Can you work these out from the model? Positions are in its coordinate system, mm. Face numbers are marked on the shaded views. A direction names the side the tool comes from. Round coordinates to 2 decimals unless told otherwise and drop trailing zeros. Write each loop counter-clockwise with the first axis right and the second up, starting at its lowest first coordinate (ties: lowest second). Pieces come first, ordered by that corner, then holes. Notation, with made-up numbers: M 89.5,56.25 L 112.5,56.25 A22 ccw 112.5,93.25 Z; hole C 33,56.25 d4. An arc over 180 degrees is marked long. Answer in a Markdown table with one row per item. Add a question column.
(1) Suppose I cut it at A-A, the plane x = 25. Write out the boundary of the cut face in (y, z) (3 decimals).
(2) If we mould it in two halves opening along X, with no side actions, what happens to the marked faces 1, 2 and 3? For each: released by +X, released by -X, zero draft, split by the parting line, or undercut.
(3) I'm going to push flat-ended pins straight in: pin 1 (5 mm diameter, centred on y = 2.5, z = 14.5, fed in from -X); pin 2 (8 mm diameter, centred on x = 25.5, z = 13.5, fed in from -Y); pin 3 (5 mm diameter, centred on y = 4.5, z = 7, fed in from -X); pin 4 (2 mm diameter, centred on x = 21, y = 2.5, fed in from +Z). Where does each tip first touch, or does it pass through?
(4) For the marked faces 4 and 5, which set-ups out of +Z, -Z, +X, -X, +Y, -Y let a thin tool reach every point of the face, with its end or its side?
(5) Suppose I cut it at B-B, the plane z = 16.75. Write out the boundary of the cut face in (x, y), then the cut area to 3 significant figures.
(6) Suppose I cut it at D-D, the plane z = 1.5. Write out the boundary of the cut face in (x, y) (3 decimals).
(7) If I drill on probe 1 along Y at (x, z) = (25, 3.25) (3 decimals); probe 2 along Z at (x, y) = (25, 0.45); probe 3 along X at (y, z) = (6.75, 18), over which ranges is the centre line in solid material (lowest first)?
(8) Suppose I cut it at C-C, the plane y = 4.25. Write out the boundary of the cut face in (x, z), then the cut area to 3 significant figures.
from build123d import *

# Parameters (mm, degrees)
PAD001_DEPTH = 1
PAD012_DEPTH = 10
SKETCH012_R  = 1.475
POCKET_DEPTH = 50


with BuildPart() as part:
    # Sketch001 → Pad001 (new body)
    with BuildSketch(Plane.XZ):
        with BuildLine():
            ThreePointArc((17.153982, 21), (25, 9.6), (32.846018, 21))
            Line((36.846018, 21), (32.846018, 21))
            Line((50, 0), (36.846018, 21))
            Line((0, 0), (50, 0))
            Line((13.153982, 21), (0, 0))
            Line((17.153982, 21), (13.153982, 21))
        make_face()
    extrude(amount=-PAD001_DEPTH)

    # Sketch011 → Pad012 (join)
    with BuildSketch(Plane.XZ):
        with BuildLine():
            ThreePointArc((14.157376, 21), (25, 6.75), (35.842624, 21))
            Line((40.842624, 21), (35.842624, 21))
            Line((50, 0), (40.842624, 21))
            Line((0, 0), (50, 0))
            Line((9.157376, 21), (0, 0))
            Line((14.157376, 21), (9.157376, 21))
        make_face()
    extrude(amount=-PAD012_DEPTH)

    # Sketch012 → Pocket (cut)
    with BuildSketch(Plane.XY):
        with Locations((25, 5)):
            Circle(SKETCH012_R)
    extrude(amount=POCKET_DEPTH, mode=Mode.SUBTRACT)


solid = part.part
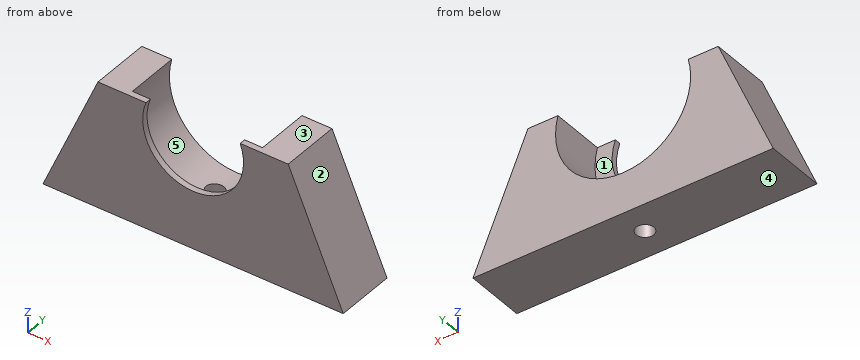
Calculated:
| question | item | result |
|---|---|---|
| 1 | outline | M 0,0 L 3.525,0 L 3.525,6.75 L 1,6.75 L 1,9.6 L 0,9.6 Z; M 6.475,0 L 10,0 L 10,6.75 L 6.475,6.75 Z |
| 2 | face 1 | undercut |
| 2 | face 2 | released by +X |
| 2 | face 3 | zero draft |
| 3 | pin 1 | x = 5.23 |
| 3 | pin 2 | y = 0 |
| 3 | pin 3 | x = 1.96 |
| 3 | pin 4 | z = 7.92 |
| 4 | face 4 | -Z, +X, -X, +Y, -Y |
| 4 | face 5 | +Y |
| 5 | outline | M 7.3,0 L 16.69,0 L 16.69,1 L 13.82,1 L 13.82,10 L 7.3,10 Z; M 33.31,0 L 42.7,0 L 42.7,10 L 36.18,10 L 36.18,1 L 33.31,1 Z |
| 5 | area | 136 mm² |
| 6 | outline | M 0.654,0 L 49.346,0 L 49.346,10 L 0.654,10 Z; hole C 25,5 d2.95 |
| 7 | probe 1 | 0 to 3.525, 6.475 to 10 |
| 7 | probe 2 | 0 to 9.6 |
| 7 | probe 3 | 7.85 to 13.75, 36.25 to 42.15 |
| 8 | outline | M 0,0 L 23.73,0 L 23.73,6.82 A11.25 cw 14.16,21 L 9.16,21 Z; M 26.27,0 L 50,0 L 40.84,21 L 35.84,21 A11.25 cw 26.27,6.82 Z |
| 8 | area | 575 mm² |
